from build123d import *

# Parameters (mm, degrees)
SKETCH1_W           = 455
SKETCH1_H           = 330
BOSS_EXTRUDE1_DEPTH = 45
SHELL1_T            = -5


with BuildPart() as part:
    # Sketch1 → Boss-Extrude1 (new, symmetric)
    with BuildSketch(Plane(origin=(0, 0, 0), x_dir=(1, 0, 0), z_dir=(0, 1, 0))):
        Rectangle(SKETCH1_W, SKETCH1_H)
    extrude(amount=BOSS_EXTRUDE1_DEPTH, both=True)

    # Shell1
    shell1_openings = [part.faces().sort_by_distance(p)[0] for p in [
        (0, 45, 0),
    ]]
    offset(amount=SHELL1_T, openings=shell1_openings, kind=Kind.INTERSECTION)


solid = part.part
Work out the finished part from the listing and answer in its coordinate system (mm). A direction names the side the tool comes from. Give positions to 0.01 mm unless a question says otherwise; leave off trailing zeros. Loops run counter-clockwise (first coordinate to the right, second up) from the corner with the lowest first, then second, coordinate; pieces in that order, holes last. Notation, with made-up numbers: (52, 89) -> (89, 89) arc R9 ccw to (89, 103) -> close; hole circle Ø9 at (22.25, 71.5). An arc over 180 degrees is marked (long way). Use a Markdown table: item, result. Add a question column.
1) The part is cut by section B-B, the plane y = 30.5. Determine the outline of the cut face in (x, z), plus the area to 3 significant figures.
2) For a pull along X with two mould halves and no side action, classify faces 1 (the flat face through (222.5, 3, 2)), 2 (the flat face through (-227.5, 1, 2)), 3 (the flat face through (-3, 1, -165)), 4 (the flat face through (227.5, 1, 2)) as +X half, -X half, draft (parallel to the pull), parting line (faces both ways), or undercut.
3) This flat-tipped pin is pushed along its axis until it touches: P1, Ø3, axis at x = 1.5, z = -131, coming from the +Y side. Where does it stop, or does it pass through?
4) The part is cut by section C-C, the plane x = 174. Determine the outline of the cut face in (y, z).
5) The part is cut by section A-A, the plane z = -56. Determine the outline of the cut face in (x, y), plus the area to 4 significant figures.
6) Which of the six approach directions +Z, -Z, +X, -X, +Y, -Y give full straight-line access (tool end or side, diameter ignored) to faces 5 (the flat face through (-3, 1, 165)), 6 (the flat face through (-3, -40, -2))?
7) Consider line 1 along Z through (x, y) = (167, -8.5); line 2 along X through (y, z) = (-36, 117.5); line 3 along Y through (x, z) = (206, 41). Determine where each line is inside the solid, lowest interval first.
Reported:
| question | item | result |
|---|---|---|
| 1 | outline | (-227.5, -165) -> (227.5, -165) -> (227.5, 165) -> (-227.5, 165) -> close; hole (-222.5, -160) -> (222.5, -160) -> (222.5, 160) -> (-222.5, 160) -> close |
| 1 | area | 7,750 mm^2 |
| 2 | face 1 | undercut |
| 2 | face 2 | -X half |
| 2 | face 3 | draft |
| 2 | face 4 | +X half |
| 3 | P1 | stops at y = -40 |
| 4 | outline | (-45, -165) -> (45, -165) -> (45, -160) -> (-40, -160) -> (-40, 160) -> (45, 160) -> (45, 165) -> (-45, 165) -> close |
| 5 | outline | (-227.5, -45) -> (227.5, -45) -> (227.5, 45) -> (222.5, 45) -> (222.5, -40) -> (-222.5, -40) -> (-222.5, 45) -> (-227.5, 45) -> close |
| 5 | area | 3,125 mm^2 |
| 6 | face 5 | +Z, +X, -X, +Y, -Y |
| 6 | face 6 | +Y |
| 7 | line 1 | z = -165 to -160, 160 to 165 |
| 7 | line 2 | x = -227.5 to -222.5, 222.5 to 227.5 |
| 7 | line 3 | y = -45 to -40 |
